Design review of the part shown in the three views and the two pictorial views. Dimensions are in mm from the part's minimum x, y and z. A direction names the side the tool comes from. Give positions to 0.01 mm unless a question says otherwise; leave off trailing zeros. Loops run counter-clockwise (first coordinate to the right, second up) from the corner with the lowest first, then second, coordinate; pieces in that order, holes last. Notation, with made-up numbers: (12.25, 6) - (66.25, 6) arc R25 ccw to (66.25, 35) - close; hole circle Ø5 at (58.25, 27). An arc over 180 degrees is marked (long way). Put each result on its own line as item: value. Start each with the question number.
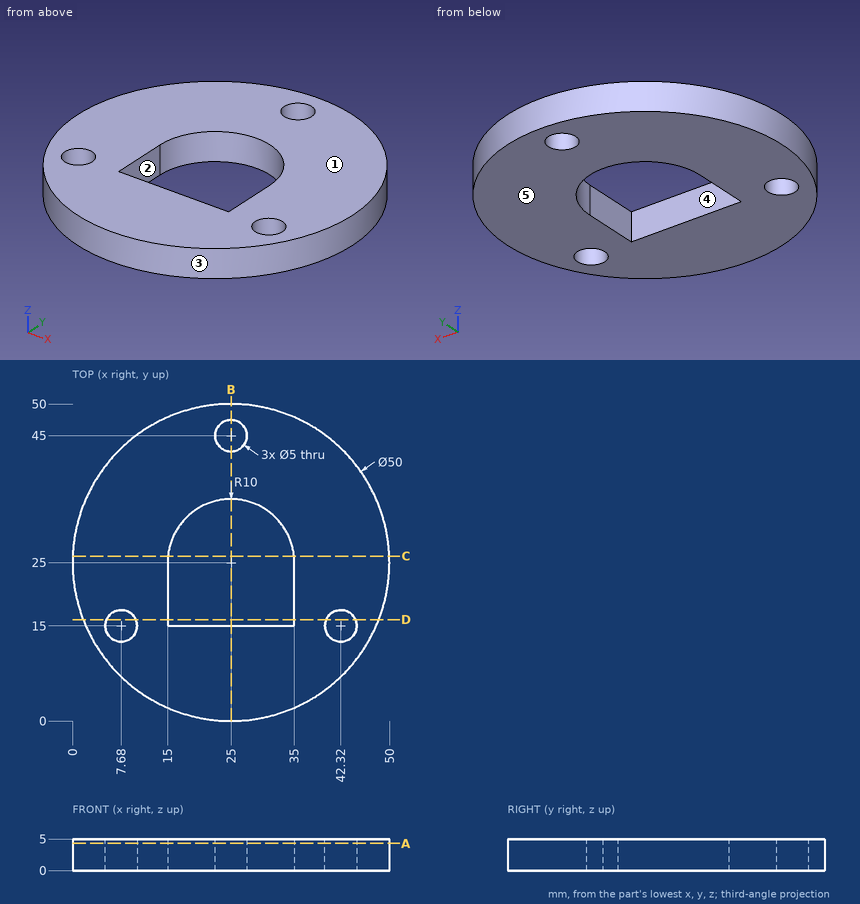
1) Take a section at D-D on y = 16. State the section outline as (x, z) points.
2) Take a section at C-C on y = 26. State the section outline as (x, z) points.
3) Take a section at A-A on z = 4.3. State the section outline as (x, y) points.
4) Wall thickness on probe 1 along Y at (x, z) = (25, 1.05); probe 2 along X at (y, z) = (18.5, 1); probe 3 along Y at (x, z) = (28, 4.45): over which ranges is each line inside the solid? List them lowest first.
5) Insertion check: P1, Ø2.5, axis at y = 17.5, z = 3.5, coming from the -X side; P2, Ø1.5, axis at y = 21.5, z = 2, coming from the +X side; P3, Ø4, axis at x = 42.32, y = 15, coming from the -Z side; P4, Ø1, axis at x = 16, z = 2.5, coming from the -Y side. Each pin has a flat end and moves straight along its axis. Give the tip position at first contact, or say it passes through.
6) Machinability: for the marked faces 1 and 2, which of the approach directions +Z, -Z, +X, -X, +Y, -Y give a long, thin tool a straight path to every point of the face, cutting with its end or side? Answer none if there is none.
7) Mouldability with a two-part tool opening along Y and no side actions: class the marked faces 3, 4 and 5 as released by +Y, released by -Y, zero draft, split by the parting line, or undercut.
8) Take a section at B-B on x = 25. State the section outline as (y, z) points.
Answers follow:
1. outline: (1.68, 0) - (5.39, 0) - (5.39, 5) - (1.68, 5) - close; (9.97, 0) - (15, 0) - (15, 5) - (9.97, 5) - close; (35, 0) - (40.03, 0) - (40.03, 5) - (35, 5) - close; (44.61, 0) - (48.32, 0) - (48.32, 5) - (44.61, 5) - close
2. outline: (0.02, 0) - (15.05, 0) - (15.05, 5) - (0.02, 5) - close; (34.95, 0) - (49.98, 0) - (49.98, 5) - (34.95, 5) - close
3. outline: circle Ø50 at (25, 25); hole circle Ø5 at (7.68, 15); hole (15, 15) - (35, 15) - (35, 25) arc R10 ccw to (15, 25) - close; hole circle Ø5 at (25, 45); hole circle Ø5 at (42.32, 15)
4. probe 1: 0 to 15, 35 to 42.5, 47.5 to 50
4. probe 2: 0.86 to 15, 35 to 49.14
4. probe 3: 0.18 to 15, 34.54 to 49.82
5. P1: x = 0.79
5. P2: x = 49.85
5. P3: through
5. P4: y = 1.49
6. face 1: +Z, +X, -X, +Y, -Y
6. face 2: +Z, -Z
7. face 3: split by the parting line
7. face 4: undercut
7. face 5: zero draft
8. outline: (0, 0) - (15, 0) - (15, 5) - (0, 5) - close; (35, 0) - (42.5, 0) - (42.5, 5) - (35, 5) - close; (47.5, 0) - (50, 0) - (50, 5) - (47.5, 5) - close
